For this review, take the finished solid that the model builds, in its own axes (mm). A direction names the side the tool comes from. Give positions to 0.01 mm unless a question says otherwise; leave off trailing zeros. Order: outer loops, then holes, each group sorted by start corner. A loop starts at its lowest first (then second) coordinate and runs counter-clockwise, first axis right, second up.
Item 1: Consider section A-A (z = -136). Give the boundary of the cut face in (x, y), plus the area to 3 significant figures.
Item 2: Consider section C-C (x = -74). Give the boundary of the cut face in (y, z), plus the area to 3 significant figures.
Item 3: For P1, Ø10, axis at x = -31.5, y = 128.5, coming from the -Z side; P2, Ø3, axis at x = -31, y = 51, coming from the +Z side; P3, Ø10, axis at x = -21.5, y = -110.5, coming from the +Z side, all flat-tipped, find the tip position at first contact; note any pin that passes through.
Item 4: Consider section B-B (y = -48). Give the boundary of the cut face in (x, z).
Item 5: For probe 1 along X at (y, z) = (-175, -41); probe 2 along Z at (x, y) = (-124, 175); probe 3 along X at (y, z) = (200, -94), list the stretches that pass through material, from the lowest coordinate up.
Item 6: Machinability: for faces 4 (the flat face through (-190, -4, -157)), 5 (the flat face through (-190, -4, -42)), 6 (the flat face through (-7, -4, -200)), which of the approach directions +Z, -Z, +X, -X, +Y, -Y give a long, thin tool a straight path to every point of the face, cutting with its end or side? Answer none if there is none.
Item 7: The part is to be moulded in two halves that separate along X. For faces 1 (the flat face through (-205, -4, -101)), 2 (the flat face through (-8, -4, 0)), 3 (the flat face through (-15, -4, -158)), say which applies: released by +X, released by -X, zero draft, split by the parting line, or undercut.
Autodesk Inventor part; units mm, degrees
ref_plane "YZ Plane" through (0, 0, 0) normal (1, 0, 0) x (0, 1, 0)
ref_plane "XZ Plane" through (0, 0, 0) normal (0, 1, 0) x (-1, 0, 0)
ref_plane "XY Plane" through (0, 0, 0) normal (0, 0, 1) x (1, 0, 0)
sketch "Szkic1" plane through (0, 0, 0) normal (0, 1, 0) x (-1, 0, 0)
  line L0 (0, 0) -> (0, -200)
  line L1 (0, -200) -> (15, -200)
  line L2 (15, -200) -> (15, -105)
  line L3 (15, -105) -> (190, -105)
  line L4 (190, -105) -> (190, -200)
  line L5 (190, -200) -> (205, -200)
  line L6 (205, -200) -> (205, 0)
  line L7 (205, 0) -> (190, 0)
  line L8 (190, 0) -> (190, -95)
  line L9 (190, -95) -> (15, -95)
  line L10 (15, -95) -> (15, 0)
  line L11 (15, 0) -> (0, 0)
  line L12 (15, 0) -> (0, 0)
  dimension "d0" = 200
  dimension "d1" = 15
  dimension "d2" = 95
  dimension "d3" = 175
  dimension "d4" = 15
  dimension "d5" = 95
extrude "Wyciągnięcie proste1" add sketch "Szkic1" along normal mid plane 500
fillet "Zaokrąglenie2" radius 10 4 edges at (-190, 0, -105) (-15, 0, -105) (-15, 0, -95) (-190, 0, -95)
properties part number "Pierwszy projekt"
Resolved:
1. outline: (-205, -250) - (-190, -250) - (-190, 250) - (-205, 250) - close; (-15, -250) - (0, -250) - (0, 250) - (-15, 250) - close
1. area: 15,000 mm2
2. outline: (-250, -105) - (250, -105) - (250, -95) - (-250, -95) - close
2. area: 5,000 mm2
3. P1: stops at z = -105
3. P2: stops at z = -95
3. P3: stops at z = -90.27
4. outline: (-205, -200) - (-190, -200) - (-190, -115) arc R10 cw to (-180, -105) - (-25, -105) arc R10 cw to (-15, -115) - (-15, -200) - (0, -200) - (0, 0) - (-15, 0) - (-15, -85) arc R10 cw to (-25, -95) - (-180, -95) arc R10 cw to (-190, -85) - (-190, 0) - (-205, 0) - close
5. probe 1: x = -205 to -190, -15 to 0
5. probe 2: z = -105 to -95
5. probe 3: x = -205 to -184.36, -20.64 to 0
6. face 4: -Z, +Y, -Y
6. face 5: +Z, +Y, -Y
6. face 6: -Z, +X, -X, +Y, -Y
7. face 1: released by -X
7. face 2: zero draft
7. face 3: undercut
